Autodesk Inventor part; units mm, degrees
ref_plane "YZ Plane" through (0, 0, 0) normal (1, 0, 0) x (0, 1, 0)
ref_plane "XZ Plane" through (0, 0, 0) normal (0, 1, 0) x (-1, 0, 0)
ref_plane "XY Plane" through (0, 0, 0) normal (0, 0, 1) x (1, 0, 0)
sketch "Sketch1" plane through (0, 0, 0) normal (0, 1, 0) x (-1, 0, 0)
  line L0 (0, 0) -> (12.7, 0)
  line L1 (12.7, 0) -> (12.7, -47.625)
  line L2 (12.7, -47.625) -> (0, -47.625)
  line L3 (0, -47.625) -> (0, 0)
  line L4 (6.35, 0) -> (6.35, -6.35)
  circle A0 centre (6.35, -6.35) radius 2.1082
  line L5 (6.35, -6.35) -> (6.35, -19.05)
  circle A1 centre (6.35, -19.05) radius 2.1082
  line L6 (6.35, -19.05) -> (6.35, -53.975)
  line L7 (6.35, -53.975) -> (12.7, -53.975)
  circle A2 centre (12.7, -53.975) radius 2.1082
  line L8 (12.7, -53.975) -> (12.7, -60.325)
  arc A3 (12.7, -60.325) -> (12.7, -47.625) centre (12.7, -53.975) ccw
  line L9 (0, -47.625) -> (0, -53.975)
  line L10 (12.7, -60.325) -> (3.175, -60.325)
  line L11 (0, -57.15) -> (0, -53.975)
  arc A4 (0, -57.15) -> (3.175, -60.325) centre (3.175, -57.15) ccw
  dimension "d0" = 12.7
  dimension "d1" = 6.35
  dimension "d2" = 4.2164
  dimension "d3" = 47.625
  dimension "d4" = 12.7
  dimension "d5" = 34.925
  dimension "d6" = 6.35
  dimension "d7" = 4.2164
  dimension "d8" = 6.35
  dimension "d9" = 3.175
extrude "Extrusion1" add sketch "Sketch1" along normal blind 6.35 contours L0 L4 A0 L5 A1 L6 L2 L3 | L0 L1 L2 L6 A1 L5 A0 L4 | L2 L6 L7 A2 L8 L10 A4 L11 L9 | L2 A3 L8 A2 L7 L6
sketch "Sketch2" plane through (0, 6.35, 0) normal (0, 1, 0) x (1, 0, 0)
  point P0 (0, 0)
properties part number "wing mount printed version" material "Aluminum 6061"
Design review of the part built by this model. Coordinates are the model's own, in mm. A direction names the side the tool comes from. Coordinates: 2 decimals unless noted, no trailing zeros. Order: outer loops, then holes, each group sorted by start corner. A loop starts at its lowest first (then second) coordinate and runs counter-clockwise, first axis right, second up.
Item 1: Take a section at B-B, the plane z = -6.35. Write out the cut boundary in (x, y), then the cut area to 3 significant figures.
Item 2: For faces 1 (the cylindrical face through (-6.08, 3.13, -8.44)), 2 (the flat face through (-12.7, 3, -23)), list the 3-axis set-ups (+Z, -Z, +X, -X, +Y, -Y) from which the entire face can be reached by the end or side of a thin tool; tool diameter is ignored.
Item 3: For line 1 (Z direction, x = -6.35, y = 3.75) (3 decimals); line 2 (X direction, y = 2.25, z = -19.05); line 3 (Z direction, x = -7.5, y = 5.5) (3 decimals), list the stretches that pass through material, from the lowest coordinate up.
Item 4: Take a section at D-D, the plane y = 4.75. Write out the cut boundary in (x, z) (3 decimals), then the cut area to 3 significant figures.
Item 5: Take a section at C-C, the plane x = -13.5. Write out the cut boundary in (y, z), then the cut area to 3 significant figures.
Item 6: For pin 1 Ø4 at (x, z) = (-6.35, -6.35) entering from +Y, flat-tipped, find the tip position at first contact; note if it passes through.
Item 7: The part is to be moulded in two halves that separate along Z. For faces 3 (the cylindrical face through (-12.243, 3.131, -51.917)), 4 (the cylindrical face through (-0.955, 3.131, -59.42)), 5 (the flat face through (-6, 3, 0)), say which applies: pulls with the +Z half, pulls with the -Z half, needs draft (parallel to the pull), parting line crosses it, or undercut.
Item 8: Take a section at A-A, the plane x = -6.35. Write out the cut boundary in (y, z) (3 decimals).
The answers:
1. outline: (-12.7, 0) - (-8.46, 0) - (-8.46, 6.35) - (-12.7, 6.35) - close; (-4.24, 0) - (0, 0) - (0, 6.35) - (-4.24, 6.35) - close
1. area: 53.9 mm2
2. face 1: +Y, -Y
2. face 2: +Z, -X, +Y, -Y
3. line 1: z = -60.325 to -21.158, -16.942 to -8.458, -4.242 to 0
3. line 2: x = -12.7 to -8.46, -4.24 to 0
3. line 3: z = -60.325 to -20.817, -17.283 to -8.117, -4.583 to 0
4. outline: (-12.7, -60.325) - (-3.175, -60.325) arc R3.175 ccw to (0, -57.15) - (0, 0) - (-12.7, 0) - (-12.7, -47.625) arc R6.35 ccw to start; hole circle Ø4.216 at (-12.7, -53.975); hole circle Ø4.216 at (-6.35, -19.05); hole circle Ø4.216 at (-6.35, -6.35)
4. area: 785 mm2
5. outline: (0, -60.27) - (6.35, -60.27) - (6.35, -55.93) - (0, -55.93) - close; (0, -52.02) - (6.35, -52.02) - (6.35, -47.68) - (0, -47.68) - close
5. area: 55.2 mm2
6. pin 1: passes through
7. face 3: undercut
7. face 4: pulls with the -Z half
7. face 5: pulls with the +Z half
8. outline: (0, -60.325) - (6.35, -60.325) - (6.35, -21.158) - (0, -21.158) - close; (0, -16.942) - (6.35, -16.942) - (6.35, -8.458) - (0, -8.458) - close; (0, -4.242) - (6.35, -4.242) - (6.35, 0) - (0, 0) - close
